Here's how the part is built. I have some questions about the finished solid (model axes, mm). A direction names the side the tool comes from. Coordinates: 2 decimals unless noted, no trailing zeros. Order: outer loops, then holes, each group sorted by start corner. A loop starts at its lowest first (then second) coordinate and runs counter-clockwise, first axis right, second up. Notation, with made-up numbers: (-11.5, 10) - (24.5, 10) arc R28 cw to (24.5, 28) - close; hole circle Ø4 at (-22, 48). An arc over 180 degrees is marked (long way). Answer in a Markdown table with one row per item. Add a question column.
Item 1: Thinking about a two-plate mould opening in X: for faces 4 (the flat face through (-33, 4, -14)), 5 (the cylindrical face through (-22.62, 10.2, -18.92)), 6 (the cylindrical face through (-8.825, 2.218, -6.036)), 7 (the flat face through (-8, 2, 0)), which applies, +X half, -X half, draft (parallel to the pull), parting line (faces both ways), or undercut?
Item 2: I want a section at C-C (z = -7.5). Please give me the cut outline in (x, y).
Item 3: I want a section at B-B (y = 6). Please give me the cut outline in (x, z).
Item 4: I want a section at D-D (y = 8.5). Please give me the cut outline in (x, z), plus the area to 3 significant figures.
Item 5: Will these pins go through, and if not, where does the flat tip stop? pin 1 Ø12 at (x, z) = (-5.5, -9.5) entering from +Y; pin 2 Ø4 at (x, z) = (-6.5, -17) entering from +Y; pin 3 Ø4 at (x, y) = (-12, 4.5) entering from +Z.
Item 6: If I drill on line 1 along Z through (x, y) = (-27.5, 4); line 2 along X through (y, z) = (2.5, -7.5); line 3 along Z through (x, y) = (-8.5, 2.65), over which ranges is the centre line in solid material (lowest first)? Write a range as from..to.
Item 7: I want a section at A-A (x = -8.5). Please give me the cut outline in (y, z).
Item 8: On a 3-axis mill with a long thin cutter (end or side, diameter ignored), from which of +Z, -Z, +X, -X, +Y, -Y can I reach the whole of each face in a straight line? I mean faces 1 (the cylindrical face through (-32.38, 10.2, -1.08)), 2 (the flat face through (-9, 6, -32)), 3 (the flat face through (0, 3, -16)). Say none if no direction works.
```python
from build123d import *

# Parameters (mm, degrees)
SKETCH1_W                = 33
SKETCH1_H                = 33
BOSS_EXTRUDE1_DEPTH      = 7
SKETCH2_W                = 15
SKETCH2_H                = 32
CUT_EXTRUDE1_DEPTH       = 2.5
SKETCH4_W                = 17
SKETCH4_H                = 5
BOSS_EXTRUDE3_DEPTH      = 7
SKETCH3_R                = 5
SKETCH3_R_2              = 2.5
BOSS_EXTRUDE4_DEPTH      = 6.5
CUT_EXTRUDE4_START       = -7
CUT_EXTRUDE4_OUTLINE_R   = 2.5
CUT_EXTRUDE4_OUTLINE_R_2 = 1.5
CUT_EXTRUDE4_DEPTH       = 7


# Read off the part's stored shape, not the designer's step: Cut-Extrude4
with BuildPart() as part:
    # Sketch1 → Boss-Extrude1 (new body)
    with BuildSketch(Plane(origin=(0, 0, 0), x_dir=(1, 0, 0), z_dir=(0, 1, 0))):
        with Locations((-16.5, 16.5)):
            Rectangle(SKETCH1_W, SKETCH1_H)
    extrude(amount=BOSS_EXTRUDE1_DEPTH)

    # Sketch2 → Cut-Extrude1 (cut)
    with BuildSketch(Plane(origin=(0, 7, 0), x_dir=(1, 0, 0), z_dir=(0, 1, 0))):
        with Locations((-8.5, 16)):
            Rectangle(SKETCH2_W, SKETCH2_H)
    extrude(amount=-CUT_EXTRUDE1_DEPTH, mode=Mode.SUBTRACT)

    # Sketch4 → Boss-Extrude3 (add)
    with BuildSketch(Plane(origin=(0, 7, 0), x_dir=(1, 0, 0), z_dir=(0, 1, 0))):
        with Locations((-24.5, -2.5)):
            Rectangle(SKETCH4_W, SKETCH4_H)
    extrude(amount=-BOSS_EXTRUDE3_DEPTH)

    # Sketch3 → Boss-Extrude4 (add)
    # profile 1 of 2: a face of its own
    with BuildSketch(Plane(origin=(0, 7, 0), x_dir=(1, 0, 0), z_dir=(0, 1, 0))):
        with Locations(Location((-27.5, 20, 0), (0, 0, 90))):
            Circle(SKETCH3_R)
        with Locations(Location((-27.5, 20, 0), (0, 0, 90))):
            Circle(SKETCH3_R_2, mode=Mode.SUBTRACT)
    # profile 2 of 2: a face of its own
    with BuildSketch(Plane(origin=(0, 7, 0), x_dir=(1, 0, 0), z_dir=(0, 1, 0))):
        with Locations(Location((-27.5, 0, 0), (0, 0, 270))):
            Circle(SKETCH3_R)
        with Locations(Location((-27.5, 0, 0), (0, 0, 90))):
            Circle(SKETCH3_R_2, mode=Mode.SUBTRACT)
    extrude(amount=BOSS_EXTRUDE4_DEPTH)

    # Cut-Extrude4 outline → Cut-Extrude4 (cut)
    with BuildSketch(Plane(origin=(0, 7, 0), x_dir=(1, 0, 0), z_dir=(0, 1, 0)).offset(CUT_EXTRUDE4_START)):
        with Locations((-27.5, 20)):
            Circle(CUT_EXTRUDE4_OUTLINE_R)
        with Locations((-27.5, 0)):
            Circle(CUT_EXTRUDE4_OUTLINE_R)
        with Locations((-8.5, 7.5)):
            Circle(CUT_EXTRUDE4_OUTLINE_R_2)
    extrude(amount=CUT_EXTRUDE4_DEPTH, mode=Mode.SUBTRACT)


solid = part.part
```
Values follow:
| question | item | result |
|---|---|---|
| 1 | face 4 | -X half |
| 1 | face 5 | parting line |
| 1 | face 6 | undercut |
| 1 | face 7 | draft |
| 2 | outline | (-33, 0) - (-10, 0) - (-10, 4.5) - (-16, 4.5) - (-16, 7) - (-33, 7) - close; (-7, 0) - (0, 0) - (0, 7) - (-1, 7) - (-1, 4.5) - (-7, 4.5) - close |
| 3 | outline | (-33, -33) - (0, -33) - (0, 0) - (-1, 0) - (-1, -32) - (-16, -32) - (-16, 5) - (-33, 5) - close; hole circle Ø5 at (-27.5, -20); hole circle Ø5 at (-27.5, 0) |
| 4 | outline | circle Ø10 at (-27.5, -20); circle Ø10 at (-27.5, 0); hole circle Ø5 at (-27.5, -20); hole circle Ø5 at (-27.5, 0) |
| 4 | area | 118 mm^2 |
| 5 | pin 1 | stops at y = 7 |
| 5 | pin 2 | stops at y = 4.5 |
| 5 | pin 3 | stops at z = 0 |
| 6 | line 1 | z = -33..-22.5, -17.5..-2.5, 2.5..5 |
| 6 | line 2 | x = -33..-10, -7..0 |
| 6 | line 3 | z = -33..-9, -6..0 |
| 7 | outline | (0, -33) - (7, -33) - (7, -32) - (4.5, -32) - (4.5, -9) - (0, -9) - close; (0, -6) - (4.5, -6) - (4.5, 0) - (0, 0) - close |
| 8 | face 1 | +Y |
| 8 | face 2 | +Z, +Y |
| 8 | face 3 | +Z, -Z, +X, +Y, -Y |
